Here's how the part is built. I have some questions about the finished solid (model axes, mm). Face numbers are marked on the shaded views. A direction names the side the tool comes from. Round coordinates to 2 decimals unless told otherwise and drop trailing zeros. Order: outer loops, then holes, each group sorted by start corner. A loop starts at its lowest first (then second) coordinate and runs counter-clockwise, first axis right, second up.
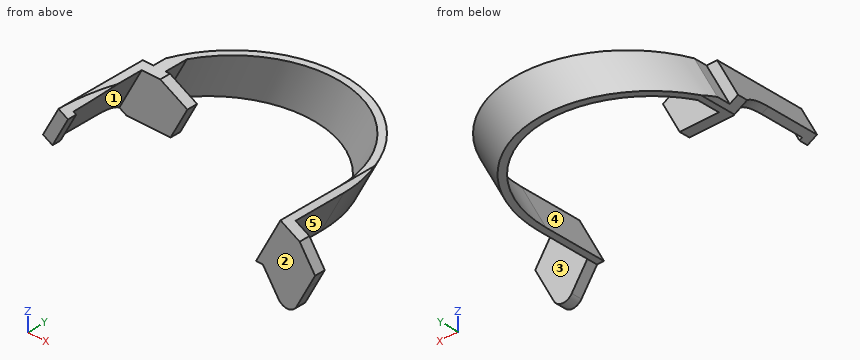
```python
from build123d import *

# Parameters (mm, degrees)
CORTE_EXTRUS_O1_DEPTH      = 51.4
CORTE_EXTRUS_O2_DEPTH      = 73.874980511
CHANFRO1_SIZE              = 10
CHANFRO1_SIZE2             = 4.694715628
ESBO_O6_W                  = 5.368395338
ESBO_O6_H                  = 18.334195556
CORTE_EXTRUS_O3_DEPTH      = 5
CORTE_EXTRUS_O3_DEPTH_BACK = 5
RESSALTO_EXTRUS_O2_DEPTH   = 3
CHANFRO2_SIZE              = 7
CHANFRO2_SIZE2             = 3.721966022
FILETE2_R                  = 3


with BuildPart() as part:
    # Varredura2: sweep along a path in Esboço2
    with BuildLine(Plane(origin=(0, 0, 0), x_dir=(1, 0, 0), z_dir=(0, 1, 0))) as varredura2_path:
        Line((0, 0), (-7.042073442, 13.244213893))
    # Esboço1<3> → Varredura2 (sweep)
    with BuildSketch(Plane.XY):
        with BuildLine():
            Line((30.5, 0), (30.5, -17.9))
            Line((30.5, -17.9), (45.5, -17.9))
            Line((45.5, -17.9), (45.5, -14.9))
            Line((45.5, -14.9), (32.5, -14.9))
            Line((32.5, -14.9), (32.5, 0))
            ThreePointArc((32.5, 0), (6.046693311, 31.932546093), (-30.25, 11.882234638))
            Line((-30.25, 11.882234638), (-30.25, 8.1))
            Line((-30.25, 8.1), (-33.3, 8.1))
            Line((-33.3, 8.1), (-33.3, -17.9))
            Line((-33.3, -17.9), (-30.8, -17.9))
            Line((-30.8, -17.9), (-29.8, -17.9))
            Line((-29.8, -17.9), (-29.8, -15.416139266))
            Line((-29.8, -15.416139266), (-30.8, -15.416139266))
            Line((-30.8, -15.416139266), (-30.8, 5.1))
            Line((-30.8, 5.1), (-26.75, 5.1))
            Line((-26.75, 5.1), (-15.5, 5.1))
            Line((-15.5, 5.1), (-15.5, 8.1))
            Line((-15.5, 8.1), (-26.75, 8.1))
            Line((-26.75, 8.1), (-26.75, 14.652218262))
            ThreePointArc((-26.75, 14.652218262), (7.562241731, 29.547631039), (30.5, 0))
        make_face()
    sweep(path=varredura2_path.line)

    # Esboço4 → Corte-extrusão1 (cut, through all)
    with BuildSketch(Plane.XZ.offset(17.9)):
        Polygon((42.193946776, -6.217781794), (30.5, 0), (45.5, 0), align=None)
    extrude(amount=-CORTE_EXTRUS_O1_DEPTH, mode=Mode.SUBTRACT)

    # Esboço5 → Corte-extrusão2 (cut, through all)
    with BuildSketch(Plane(origin=(-25.960561843, 0, 13.803475583), x_dir=(0.469471563, 0, 0.882947593), z_dir=(-0.882947593, 0, 0.469471563))):
        with BuildLine():
            Line((-30.633403041, -17.9), (-25.133403041, -17.9))
            Line((-25.133403041, -17.9), (-25.133403041, -2.9))
            ThreePointArc((-25.133403041, -2.9), (-26.599119213, 2.806356105), (-30.633403041, 7.1))
            Line((-30.633403041, 7.1), (-30.633403041, -17.9))
        make_face()
        with BuildLine():
            Line((-13.16947903, 4.679780509), (-13.16947903, -17.9))
            Line((-13.16947903, -17.9), (-15.633403041, -17.9))
            ThreePointArc((-15.633403041, -17.9), (-15.015599199, -6.543092307), (-13.16947903, 4.679780509))
        make_face()
    extrude(amount=-CORTE_EXTRUS_O2_DEPTH, mode=Mode.SUBTRACT)

    # Chanfro1
    chanfro1_edges = [part.edges().sort_by_distance(p)[0] for p in [
        (-15.5, 6.6, 0),
    ]]
    chanfro1_side = [part.faces().sort_by_distance(p)[0] for p in [
        (-23.15, 5.913055964, 0),
    ]]
    chamfer(chanfro1_edges, length=CHANFRO1_SIZE, length2=CHANFRO1_SIZE2, reference=chanfro1_side[0])

    # Esboço6 → Corte-extrusão3 (cut, two sides)
    with BuildSketch(Plane(origin=(-24.011570713, 0, 12.767178617), x_dir=(-0.469471563, 0, -0.882947593), z_dir=(0.882947593, 0, -0.469471563))) as corte_extrus_o3_sk:
        with Locations((31.085712443, 8.557015368)):
            Rectangle(ESBO_O6_W, ESBO_O6_H)
    extrude(amount=CORTE_EXTRUS_O3_DEPTH, mode=Mode.SUBTRACT)
    extrude(corte_extrus_o3_sk.sketch, amount=-CORTE_EXTRUS_O3_DEPTH_BACK, mode=Mode.SUBTRACT)

    # Esboço7 → Ressalto-extrusão2 (add)
    with BuildSketch(Plane(origin=(0, -14.9, 0), x_dir=(1, 0, 0), z_dir=(0, 1, 0))):
        Polygon((25.457926558, 13.244213893), (32.727434303, 24.021702336), (38.457926558, 13.244213893), align=None)
    extrude(amount=-RESSALTO_EXTRUS_O2_DEPTH)

    # Chanfro2
    chanfro2_edges = [part.edges().sort_by_distance(p)[0] for p in [
        (42.193946776, -16.4, -6.217781794),
    ]]
    chanfro2_side = [part.faces().sort_by_distance(p)[0] for p in [
        (36.346973388, -17.580051063, -3.108890897),
    ]]
    chamfer(chanfro2_edges, length=CHANFRO2_SIZE, length2=CHANFRO2_SIZE2, reference=chanfro2_side[0])

    # Filete2
    filete2_edges = [part.edges().sort_by_distance(p)[0] for p in [
        (32.727434303, -16.4, -24.021702336),
    ]]
    fillet(filete2_edges, radius=FILETE2_R)


solid = part.part
```
1. I need wall thicknesses on probe 1 along X at (y, z) = (27, -11.75); probe 2 along Y at (x, z) = (-24, -1); probe 3 along Y at (x, z) = (-24.5, -4.75). Which ranges of each line are inside material? Lowest first, please.
Evaluation:
probe 1: x = -24.34 to -20.43, 7.94 to 11.84
probe 2: y = 5.1 to 8.1, 19.48 to 22.48
probe 3: y = 5.1 to 8.1, 21.15 to 23.95
2. If we section it at B-B, the plane z = -15.25: Write out the boundary of the cut face in (x, y), and give its area (3 significant figures).
Evaluation:
outline: (26.81, -17.9) - (37.39, -17.9) - (37.39, -14.9) - (26.81, -14.9) - close
area: 31.7 mm2
3. If we mould it in two halves opening along X, with no side actions, what happens to the marked faces 3, 4 and 5? For each: released by +X, released by -X, zero draft, split by the parting line, or undercut.
Evaluation:
face 3: zero draft
face 4: undercut
face 5: released by +X
4. I'm going to push flat-ended pins straight in: P1, Ø6, axis at x = 5, z = -5, coming from the -Y side; P2, Ø10, axis at x = -33.5, z = -6.5, coming from the +Y side; P3, Ø1.5, axis at x = -13, z = -13.5, coming from the +Y side; P4, Ø4, axis at y = 15.5, z = -15.5, coming from the -X side. Where does each tip first touch, or does it pass through?
Evaluation:
P1: stops at y = 28.43
P2: stops at y = 21.49
P3: stops at y = 32.07
P4: passes through
5. On a 3-axis mill with a long thin cutter (end or side, diameter ignored), from which of +Z, -Z, +X, -X, +Y, -Y can I reach the whole of each face in a straight line? I mean the marked faces 1 and 2. Say none if no direction works.
Evaluation:
face 1: -Z
face 2: +Z, -Z, +X, -X, -Y
6. If we section it at A-A, the plane y = -8: Write out the boundary of the cut face in (x, z), and give its area (3 significant figures).
Evaluation:
outline: (-37.76, -8.39) - (-35.81, -9.42) - (-31.13, -0.62) - (-32.3, 0) - (-33.3, 0) - close; (23.46, -13.24) - (25.46, -13.24) - (32.06, -0.83) - (30.5, 0) - close
area: 47.5 mm2
